Check sheet for the modelled part. Datum: model origin and axes. Units: mm. A direction names the side the tool comes from. Give positions to 0.01 mm unless a question says otherwise; leave off trailing zeros. Write each loop counter-clockwise with the first axis right and the second up, starting at its lowest first coordinate (ties: lowest second). Pieces come first, ordered by that corner, then holes. Notation, with made-up numbers: M -35.5,6 L 1.5,6 A12 ccw 1.5,11 Z; hole C 50,59.5 d11. An arc over 180 degrees is marked long. One line per item, written item: value. Start each with the question number.
from build123d import *

# Parameters (mm, degrees)
F0_W         = 14.1
F0_H         = 23.5
F1_DEPTH     = 10.8
F2_W         = 8.2
F2_H         = 2.8
F2_H_2       = 8
F2_W_2       = 2.95
F3_DEPTH     = 5.8
F4_W         = 8.4
F4_H         = 5.9
F5_DEPTH     = 7.6
F6_R         = 5
F7_DEPTH     = 3.2
F8_R         = 2.7
F9_DEPTH     = 1.801
F10_T1_DEPTH = 37.4318792991
F11_R        = 1
F12_R        = 0.5


# Not quite as in the source:
# - a fillet or chamfer that OpenCascade refuses, or shapes differently, is made with other operations: its cross-section is extruded or revolved along the edge and cut away or added


with BuildPart() as f1:
    # F0 (on Top) → F1 (new body)
    with BuildSketch(Plane.XY):
        Rectangle(F0_W, F0_H)
    extrude(amount=F1_DEPTH)

    # F2 (on face) → F3 (cut)
    with BuildSketch(Plane.XY.offset(10.8)):
        with Locations((0, -5.4)):
            Rectangle(F2_W, F2_H)
        Rectangle(F2_W, F2_H_2)
        with Locations((5.575, 0)):
            Rectangle(F2_W_2, F2_H_2)
        with Locations((-5.575, 0)):
            Rectangle(F2_W_2, F2_H_2)
        with Locations((0, 5.4)):
            Rectangle(F2_W, F2_H)
    extrude(amount=-F3_DEPTH, mode=Mode.SUBTRACT)

    # F4 (on face) → F5 (cut)
    with BuildSketch(Plane(origin=(0, 0, 0), x_dir=(1, 0, 0), z_dir=(0, 0, -1))):
        with Locations((0, -8.8)):
            Rectangle(F4_W, F4_H)
        with Locations((0, 8.8)):
            Rectangle(F4_W, F4_H)
    extrude(amount=-F5_DEPTH, mode=Mode.SUBTRACT)

    # F6 (on face) → F7 (cut)
    with BuildSketch(Plane.XY.offset(5)):
        Circle(F6_R)
    extrude(amount=-F7_DEPTH, mode=Mode.SUBTRACT)

    # F8 (on face) → F9 (cut, through all)
    with BuildSketch(Plane.XY.offset(1.8)):
        Circle(F8_R)
    extrude(amount=-F9_DEPTH, mode=Mode.SUBTRACT)

    # F10: fillet of radius 7 on 2 edges, made by hand

    # F10_s2 → F10_t1 (cut)
    with BuildSketch(Plane.YZ.offset(-24.2909396496)):
        with BuildLine():
            ThreePointArc((-10.8963758598, 10.8), (-6.3908237294, 9.1572380944), (-4, 5))
            Line((-4, 5), (-4, 10.8))
            Line((-4, 10.8), (-10.8963758598, 10.8))
        make_face()
        with BuildLine():
            ThreePointArc((10.8963758598, 10.8), (6.3908237294, 9.1572380944), (4, 5))
            Line((4, 5), (4, 10.8))
            Line((4, 10.8), (10.8963758598, 10.8))
        make_face()
    extrude(amount=F10_T1_DEPTH, mode=Mode.SUBTRACT)

    # F11
    f11_edges = [f1.edges().sort_by_distance(p)[0] for p in [
        (7.05, -11.75, 5.4),
        (-7.05, -11.75, 5.4),
        (7.05, 11.75, 5.4),
        (-7.05, 11.75, 5.4),
    ]]
    fillet(f11_edges, radius=F11_R)

    # F12
    f12_edges = [f1.edges().sort_by_distance(p)[0] for p in [
        (0, 11.75, 10.8),
        (0, -11.75, 10.8),
        (-7.05, 0, 5),
        (7.05, 0, 5),
        (7.05, -6.335055, 9.109835),
        (7.05, 6.335055, 9.109835),
        (7.047304, -10.823382, 10.79962),
        (6.703309, -11.507092, 10.8),
        (7.047304, 10.823382, 10.79962),
        (6.703309, 11.507092, 10.8),
        (-7.05, -6.335055, 9.109835),
        (-7.047304, -10.823382, 10.799619),
        (-7.05, 6.335055, 9.109835),
        (-7.047304, 10.823382, 10.79962),
        (-6.703309, -11.507092, 10.8),
        (-6.703309, 11.507092, 10.8),
    ]]
    fillet(f12_edges, radius=F12_R)


solid = f1.part
1) Material ranges on L1, parallel to Y at x = 0, z = 4.15; L2, parallel to X at y = -10.25, z = 4.75; L3, parallel to Y at x = 0, z = 1.4, recorded low to high. Write a range as from..to.
2) Gauge pin test, flat ends, axial feed: pin 1 (6.5 mm diameter, centred on x = 0, y = -10, fed in from -Z); pin 2 (5 mm diameter, centred on x = -2, y = 6, fed in from +Z); pin 3 (2 mm diameter, centred on x = -3, z = 5.5, fed in from +Y). Record the tip position at first contact, or that the pin passes through.
3) Tool access check on faces 4 (the flat face through (-4.5, 2.7, 5)), 5 (the flat face through (4.2, 9, 4)), 6 (the cylindrical face through (-0.092, 7.333, 9.825)). Record the directions out of +Z, -Z, +X, -X, +Y, -Y that give a thin tool (end or side, any length) a straight path to the whole face; none if there is none.
4) Cross-section at D-D (y = 3). Record the boundary of the cut face in (x, z), plus the area to 3 significant figures.
5) Cross-section at B-B (y = 0). Record the boundary of the cut face in (x, z).
6) Cross-section at A-A (x = 0). Record the boundary of the cut face in (y, z).
7) Cross-section at C-C (z = 1.25). Record the boundary of the cut face in (x, y).
8) Draft check along X on faces 1 (the flat face through (0, 11.75, 9)), 2 (the flat face through (0, -5.85, 2)), 3 (the cylindrical face through (-6.765, -11.449, 5.222)). Enter one of: released by +X, released by -X, zero draft, split by the parting line, or undercut.
Data:
1. L1: y = -5.85..-5, 5..5.85
1. L2: x = -7.05..-4.2, 4.2..7.05
1. L3: y = -5.85..-2.7, 2.7..5.85
2. pin 1: stops at z = 7.6
2. pin 2: stops at z = 10.38
2. pin 3: stops at y = 5.85
3. face 4: +Z
3. face 5: -Z, +Y
3. face 6: +Z, +X, -X
4. outline: M -7.05,0 L 7.05,0 L 7.05,4.5 A0.5 ccw 6.55,5 L 4,5 L 4,1.8 L -4,1.8 L -4,5 L -6.55,5 A0.5 ccw -7.05,4.5 Z
4. area: 44.8 mm2
5. outline: M -7.05,0 L -2.7,0 L -2.7,1.8 L -5,1.8 L -5,5 L -6.55,5 A0.5 ccw -7.05,4.5 Z; M 2.7,0 L 7.05,0 L 7.05,4.5 A0.5 ccw 6.55,5 L 5,5 L 5,1.8 L 2.7,1.8 Z
6. outline: M -11.75,7.6 L -6.8,7.6 L -6.8,9.48 A7 ccw -10.9,10.8 L -11.25,10.8 A0.5 ccw -11.75,10.3 Z; M -5.85,0 L -2.7,0 L -2.7,1.8 L -5,1.8 L -5,5 L -5.85,5 Z; M 2.7,0 L 5.85,0 L 5.85,5 L 5,5 L 5,1.8 L 2.7,1.8 Z; M 6.8,7.6 L 11.75,7.6 L 11.75,10.3 A0.5 ccw 11.25,10.8 L 10.9,10.8 A7 ccw 6.8,9.48 Z
7. outline: M -7.05,-10.75 A1 ccw -6.05,-11.75 L -4.2,-11.75 L -4.2,-5.85 L 4.2,-5.85 L 4.2,-11.75 L 6.05,-11.75 A1 ccw 7.05,-10.75 L 7.05,10.75 A1 ccw 6.05,11.75 L 4.2,11.75 L 4.2,5.85 L -4.2,5.85 L -4.2,11.75 L -6.05,11.75 A1 ccw -7.05,10.75 Z; hole C 0,0 d5.4
8. face 1: zero draft
8. face 2: undercut
8. face 3: released by -X
